Study the drawing (mm; zero at the part's minimum x, y, z) and answer. Round coordinates to 2 decimals unless told otherwise and drop trailing zeros. Order: outer loops, then holes, each group sorted by start corner. A loop starts at its lowest first (then second) coordinate and runs counter-clockwise, first axis right, second up. Notation, with made-up numbers: (68.5, 19) - (112.5, 19) arc R27 cw to (112.5, 56) - close; hole circle Ø5 at (39.25, 42.5). An arc over 180 degrees is marked (long way). Put each result on its own line as item: value.
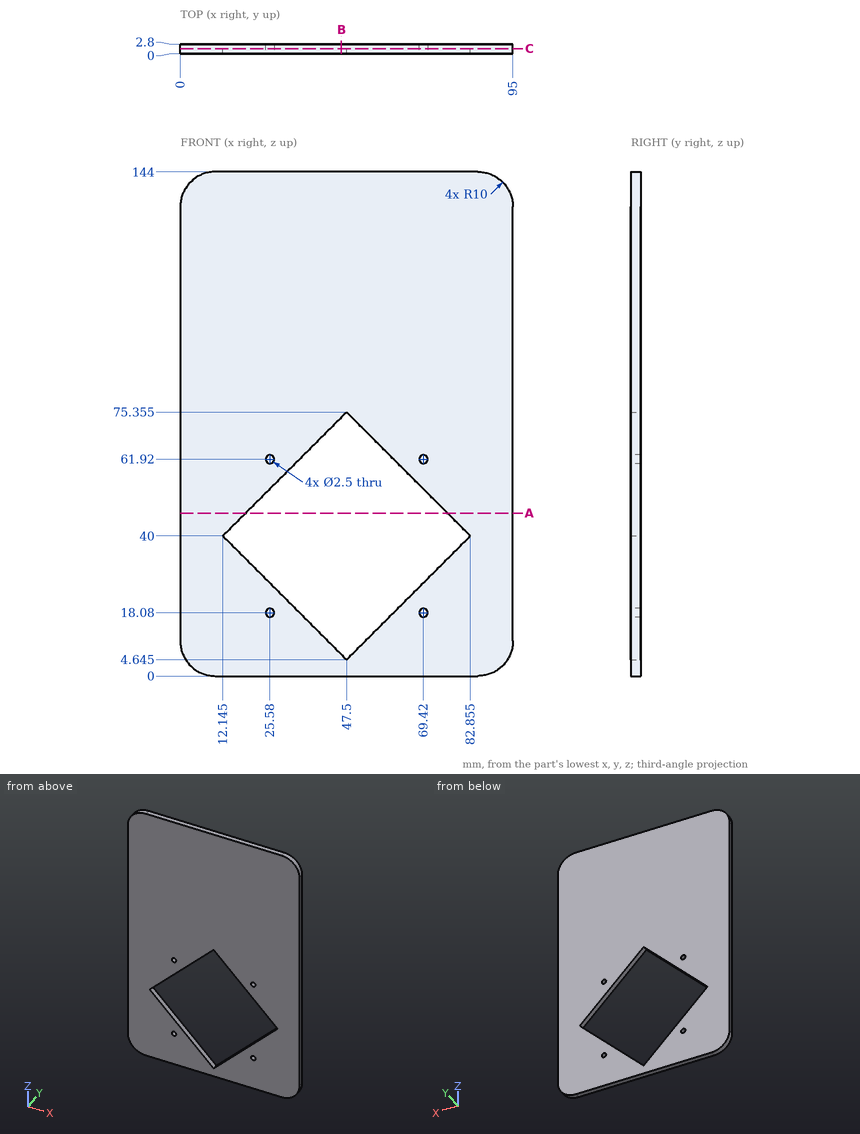
1) A cutting plane is placed at B-B on x = 46. Write down the section's boundary in (y, z) (1 decimal), then the cut area to 3 significant figures.
Findings below:
outline: (0, 0) - (2.8, 0) - (2.8, 6.1) - (0, 6.1) - close; (0, 73.9) - (2.8, 73.9) - (2.8, 144) - (0, 144) - close
area: 214 mm2
2) A cutting plane is placed at C-C on y = 1.5. Give the number of separate pieces and of enclosed holes in the cut face, then the cut area to 3 significant figures.
Findings below:
separate pieces: 1
enclosed holes: 5
area: 11,100 mm2
3) A cutting plane is placed at A-A on z = 46.5. Write down the section's boundary in (x, y) (1 decimal).
Findings below:
outline: (0, 0) - (18.6, 0) - (18.6, 2.8) - (0, 2.8) - close; (76.4, 0) - (95, 0) - (95, 2.8) - (76.4, 2.8) - close
4) Straight lines are drawn through the part: L1, parallel to Z at x = 22, y = 2.2 (1 decimal); L2, parallel to X at y = 1.3, z = 11.5 (1 decimal); L3, parallel to Z at x = 31, y = 0.55 (1 decimal). For each, find the intervals that lie inside material, in ascending order. Write a range as from..to.
Findings below:
L1: z = 0..30.1, 49.9..144
L2: x = 0..40.6, 54.4..95
L3: z = 0..21.1, 58.9..144
